```python
from build123d import *

# Parameters (mm, degrees)
F0_R     = 14
F0_R_2   = 8
F1_DEPTH = 18.5
F3_START = -5.25
F2_R     = 16.723627754
F2_R_2   = 13.5
F3_DEPTH = 1.6
F5_START = -5.25
F4_R     = 14
F4_R_2   = 13.5
F5_DEPTH = 1.6
F6_R     = 0.5


with BuildPart() as f1:
    # F0 (on Front) → F1 (new body, symmetric)
    with BuildSketch(Plane.XZ):
        Circle(F0_R)
        Circle(F0_R_2, mode=Mode.SUBTRACT)
    extrude(amount=F1_DEPTH, both=True)

    # F2 (on face) → F3 (cut)
    with BuildSketch(Plane.XZ.offset(18.5).offset(F3_START)):
        Circle(F2_R)
        Circle(F2_R_2, mode=Mode.SUBTRACT)
    extrude(amount=-F3_DEPTH, mode=Mode.SUBTRACT)

    # F4 (on face) → F5 (cut)
    with BuildSketch(Plane(origin=(0, 18.5, 0), x_dir=(-1, 0, 0), z_dir=(0, 1, 0)).offset(F5_START)):
        Circle(F4_R)
        Circle(F4_R_2, mode=Mode.SUBTRACT)
    extrude(amount=-F5_DEPTH, mode=Mode.SUBTRACT)

    # F6
    f6_edges = [f1.edges().sort_by_distance(p)[0] for p in [
        (-14, 18.5, 0),
        (-14, -18.5, 0),
    ]]
    fillet(f6_edges, radius=F6_R)


solid = f1.part
```
Here's how the part is built. I have some questions about the finished solid (model axes, mm). A direction names the side the tool comes from. Coordinates: 2 decimals unless noted, no trailing zeros. Order: outer loops, then holes, each group sorted by start corner. A loop starts at its lowest first (then second) coordinate and runs counter-clockwise, first axis right, second up. Notation, with made-up numbers: M 4.5,-33.5 L 50.5,-33.5 A22 ccw 50.5,-10.5 Z; hole C -27,13.25 d11. An arc over 180 degrees is marked long. Answer as a JSON object with one key per item and string values. Group by question number.
(1) I need wall thicknesses on probe 1 along Z at (x, y) = (0, -1); probe 2 along X at (y, z) = (12, 0.5); probe 3 along X at (y, z) = (-13, 5.5). Which ranges of each line are inside material? Lowest first, please.
(2) Which directions (+Z, -Z, +X, -X, +Y, -Y) give clear straight access to the entire face, cutting with the end or side of a thin tool? Please do faces 1 (the face through (2.93, 12.46, -13.18)), 2 (the face through (6, -18.5, -6)).
(3) If we mould it in two halves opening along Z, with no side actions, what happens to faces 3 (the face through (-2.93, -12.46, -13.18)), 4 (the face through (6, 18.5, -6)), 5 (the face through (-1.73, 0.26, -7.81))? For each: released by +Z, released by -Z, zero draft, split by the parting line, or undercut.
(4) For pin 1 (8 mm diameter, centred on y = -12, z = 2.5, fed in from -X); pin 2 (3 mm diameter, centred on x = -9.5, y = -5, fed in from -Z); pin 3 (4 mm diameter, centred on x = 3.5, y = -3, fed in from +Z), each with a flat end and sliding along its axis, tell me the tip position at first contact or that it passes through.
(5) Suppose I cut it at A-A, the plane z = 0. Please give me the cut outline in (x, y).
(6) Suppose I cut it at C-C, the plane y = -4.5. Please give me the cut outline in (x, z).
(7) Suppose I cut it at B-B, the plane x = 0. Please give me the cut outline in (y, z).
Values found:
{
 "1": {"probe 1": "z = -14 to -8, 8 to 14", "probe 2": "x = -13.49 to -7.98, 7.98 to 13.49", "probe 3": "x = -12.33 to -5.81, 5.81 to 12.33"},
 "2": {"face 1": "none", "face 2": "+Z, -Z, +X, -X, -Y"},
 "3": {"face 3": "split by the parting line", "face 4": "zero draft", "face 5": "undercut"},
 "4": {"pin 1": "stops at x = -14", "pin 2": "stops at z = -11.49", "pin 3": "stops at z = 13.92"},
 "5": {"outline": "M -14,-18 A0.5 ccw -13.5,-18.5 L -8,-18.5 L -8,18.5 L -13.5,18.5 A0.5 ccw -14,18 L -14,13.25 L -13.5,13.25 L -13.5,11.65 L -14,11.65 L -14,-11.65 L -13.5,-11.65 L -13.5,-13.25 L -14,-13.25 Z; M 8,-18.5 L 13.5,-18.5 A0.5 ccw 14,-18 L 14,-13.25 L 13.5,-13.25 L 13.5,-11.65 L 14,-11.65 L 14,11.65 L 13.5,11.65 L 13.5,13.25 L 14,13.25 L 14,18 A0.5 ccw 13.5,18.5 L 8,18.5 Z"},
 "6": {"outline": "C 0,0 d28; hole C 0,0 d16"},
 "7": {"outline": "M -18.5,-13.5 A0.5 ccw -18,-14 L -13.25,-14 L -13.25,-13.5 L -11.65,-13.5 L -11.65,-14 L 11.65,-14 L 11.65,-13.5 L 13.25,-13.5 L 13.25,-14 L 18,-14 A0.5 ccw 18.5,-13.5 L 18.5,-8 L -18.5,-8 Z; M -18.5,8 L 18.5,8 L 18.5,13.5 A0.5 ccw 18,14 L 13.25,14 L 13.25,13.5 L 11.65,13.5 L 11.65,14 L -11.65,14 L -11.65,13.5 L -13.25,13.5 L -13.25,14 L -18,14 A0.5 ccw -18.5,13.5 Z"}
}
